```python
from build123d import *

# Parameters (mm, degrees)
F0_R     = 4.7625
F1_DEPTH = 12.065
F2_R     = 1.27
F4_D     = 0.79502


with BuildPart() as f1:
    # F0 (on Front) → F1 (new body)
    with BuildSketch(Plane.XZ):
        Circle(F0_R)
    extrude(amount=F1_DEPTH)

    # F2
    f2_edges = [f1.edges().sort_by_distance(p)[0] for p in [
        (-4.7625, -12.065, 0),
        (-4.7625, 0, 0),
    ]]
    fillet(f2_edges, radius=F2_R)

    # F4 (through all)
    with Locations(Plane(origin=(0, 0, 0), x_dir=(-1, 0, 0), z_dir=(0, 1, 0))):
        with Locations((0, 0)):
            Hole(F4_D / 2)


solid = f1.part
```
Source: CAD feature listing. Evaluate the final solid. Frame: model axes, mm. Round coordinates to 2 decimals unless told otherwise and drop trailing zeros. Loops run counter-clockwise (first coordinate to the right, second up) from the corner with the lowest first, then second, coordinate; pieces in that order, holes last.
(1) Section query B-B (x = 0). Output: boundary loops of the cut face in (y, z) (1 decimal), and give its area (3 significant figures).
From the geometry:
outline: (-12.1, -3.5) arc R1.3 ccw to (-10.8, -4.8) - (-1.3, -4.8) arc R1.3 ccw to (0, -3.5) - (0, -0.4) - (-12.1, -0.4) - close; (-12.1, 0.4) - (0, 0.4) - (0, 3.5) arc R1.3 ccw to (-1.3, 4.8) - (-10.8, 4.8) arc R1.3 ccw to (-12.1, 3.5) - close
area: 104 mm2
(2) Section query C-C (y = -2). Output: boundary loops of the cut face in (x, z) (1 decimal), and give its area (3 significant figures).
From the geometry:
outline: circle Ø9.5 at (0, 0); hole circle Ø0.8 at (0, 0)
area: 70.8 mm2
(3) Section query A-A (z = 0). Output: boundary loops of the cut face in (x, y) (1 decimal).
From the geometry:
outline: (-4.8, -10.8) arc R1.3 ccw to (-3.5, -12.1) - (-0.4, -12.1) - (-0.4, 0) - (-3.5, 0) arc R1.3 ccw to (-4.8, -1.3) - close; (0.4, -12.1) - (3.5, -12.1) arc R1.3 ccw to (4.8, -10.8) - (4.8, -1.3) arc R1.3 ccw to (3.5, 0) - (0.4, 0) - close
(4) Contact query for flat-ended pins moving along their axis: pin 1 Ø1 at (x, y) = (-3.5, -6.5) entering from -Z; pin 2 Ø3 at (y, z) = (-3, 2) entering from -X; pin 3 Ø2 at (x, y) = (-2.5, -9) entering from -Z. Output: stop coordinate, or through.
From the geometry:
pin 1: stops at z = -3.7
pin 2: stops at x = -4.74
pin 3: stops at z = -4.52
(5) Material intervals for probe 1 along Z at (x, y) = (0, -3.75); probe 2 along Z at (x, y) = (-0.25, -7.75); probe 3 along Z at (x, y) = (-3.25, -3.5), sorted ascending.
From the geometry:
probe 1: z = -4.76 to -0.4, 0.4 to 4.76
probe 2: z = -4.76 to -0.31, 0.31 to 4.76
probe 3: z = -3.48 to 3.48
